Part model, mm, in its own coordinate system. Face numbers are marked on the shaded views. A direction names the side the tool comes from. Coordinates: 2 decimals unless noted, no trailing zeros. Loops run counter-clockwise (first coordinate to the right, second up) from the corner with the lowest first, then second, coordinate; pieces in that order, holes last. Notation, with made-up numbers: (39.25, 70) - (50.25, 70) arc R30 ccw to (50.25, 108) - close; hole circle Ø6 at (-5.75, 81.25). An arc over 180 degrees is marked (long way). Answer as CSV lines item,"result".
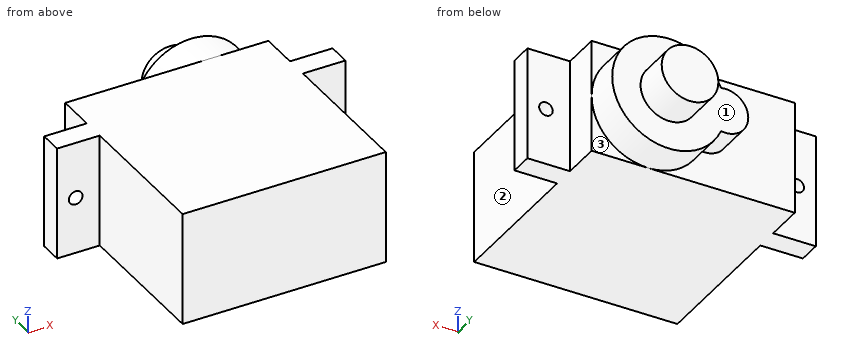
from build123d import *

# Parameters (mm, degrees)
SKETCH_1_W          = 22.4
SKETCH_1_H          = 12.5
EXTRUDE_1_DEPTH     = 22.8
EXTRUDE_START       = 16.1
SKETCH_2_W          = 31.8
SKETCH_2_H          = 12.5
EXTRUDE_2_DEPTH     = 2.5
CUT_EXTRUDE_1_REACH = 27.255
SKETCH_3_R          = 0.75
EXTRUDE_3_DEPTH     = 4
SKETCH_6_R          = 3.125
EXTRUDE_4_DEPTH     = 4.1


with BuildPart() as part:
    # 草图1 → 凸台-拉伸1 (new body)
    with BuildSketch(Plane(origin=(0, 0, 0), x_dir=(1, 0, 0), z_dir=(0, 1, 0))):
        Rectangle(SKETCH_1_W, SKETCH_1_H)
    extrude(amount=EXTRUDE_1_DEPTH)

    # 草图2 → 凸台-拉伸2 (add)
    with BuildSketch(Plane(origin=(0, 0, 0), x_dir=(1, 0, 0), z_dir=(0, 1, 0)).offset(EXTRUDE_START)):
        Rectangle(SKETCH_2_W, SKETCH_2_H)
    extrude(amount=EXTRUDE_2_DEPTH)

    # 草图3 → 切除-拉伸1 (cut, up to next)
    with BuildSketch(Plane(origin=(0, 18.6, 0), x_dir=(1, 0, 0), z_dir=(0, 1, 0)), mode=Mode.PRIVATE) as cut_extrude_1_sk1:
        with Locations(Location((-13.85, 0, 0), (0, 0, 270))):
            Circle(SKETCH_3_R)
    cut_extrude_1_tool1 = extrude(cut_extrude_1_sk1.sketch, amount=-CUT_EXTRUDE_1_REACH, mode=Mode.PRIVATE) & part.part
    # 草图3 → 切除-拉伸1 (cut, up to next)
    with BuildSketch(Plane(origin=(0, 18.6, 0), x_dir=(1, 0, 0), z_dir=(0, 1, 0)), mode=Mode.PRIVATE) as cut_extrude_1_sk2:
        with Locations(Location((13.85, 0, 0), (0, 0, 270))):
            Circle(SKETCH_3_R)
    cut_extrude_1_tool2 = extrude(cut_extrude_1_sk2.sketch, amount=-CUT_EXTRUDE_1_REACH, mode=Mode.PRIVATE) & part.part
    add(cut_extrude_1_tool1.solids().sort_by_distance((-13.85, 18.6, 0))[0], mode=Mode.SUBTRACT)
    add(cut_extrude_1_tool2.solids().sort_by_distance((13.85, 18.6, 0))[0], mode=Mode.SUBTRACT)

    # 草图4 → 凸台-拉伸3 (add)
    with BuildSketch(Plane(origin=(0, 22.8, 0), x_dir=(1, 0, 0), z_dir=(0, 1, 0))):
        with BuildLine():
            ThreePointArc((-0.8, -2.449489743), (11.2, 0), (-0.8, 2.449489743))
            ThreePointArc((-0.8, 2.449489743), (-3.8, 0), (-0.8, -2.449489743))
        make_face()
    extrude(amount=EXTRUDE_3_DEPTH)

    # 草图6 → 凸台-拉伸4 (add)
    with BuildSketch(Plane(origin=(0, 26.8, 0), x_dir=(1, 0, 0), z_dir=(0, 1, 0))):
        with Locations(Location((4.95, 0, 0), (0, 0, 270))):
            Circle(SKETCH_6_R)
    extrude(amount=EXTRUDE_4_DEPTH)


solid = part.part
Q1. Saw through at B-B (x = -1.3). Give the cut face in (y, z), then the cut area to 3 significant figures.
Results:
outline,"(0, -6.25) - (22.8, -6.25) - (22.8, -2.5) - (26.8, -2.5) - (26.8, 2.5) - (22.8, 2.5) - (22.8, 6.25) - (0, 6.25) - close"
area,"305 mm^2"
Q2. Flat gauge pins, fed straight in: pin 1 (2.5 mm diameter, centred on x = 14, z = 2.5, fed in from -Y); pin 2 (1.5 mm diameter, centred on x = -12, y = 22, fed in from +Z); pin 3 (5 mm diameter, centred on x = -14, z = 3, fed in from +Y); pin 4 (1.9 mm diameter, centred on x = 9, z = -4, fed in from +Y). Where does each tip first touch, or does it go through?
Results:
pin 1,"stops at y = 16.1"
pin 2,"passes through"
pin 3,"stops at y = 18.6"
pin 4,"stops at y = 26.8"
Q3. Saw through at C-C (z = 1.5). Give the cut face in (x, y), then the cut area to 3 significant figures.
Results:
outline,"(-15.9, 16.1) - (-11.2, 16.1) - (-11.2, 0) - (11.2, 0) - (11.2, 16.1) - (15.9, 16.1) - (15.9, 18.6) - (11.2, 18.6) - (11.2, 22.8) - (11.02, 22.8) - (11.02, 26.8) - (7.69, 26.8) - (7.69, 30.9) - (2.21, 30.9) - (2.21, 26.8) - (-3.3, 26.8) - (-3.3, 22.8) - (-11.2, 22.8) - (-11.2, 18.6) - (-15.9, 18.6) - close"
area,"614 mm^2"
Q4. Which spindle directions (+Z, -Z, +X, -X, +Y, -Y) get a long thin tool onto all of the face, cutting with end or side? Do the marked faces 1, 2 and 3. Say none if no direction does.
Results:
face 1,"+Y"
face 2,"+Z, -Z, +X, -Y"
face 3,"-Z, +X, +Y"
Q5. Saw through at A-A (x = -13.85). Give the cut face in (y, z).
Results:
outline,"(16.1, -6.25) - (18.6, -6.25) - (18.6, -0.75) - (16.1, -0.75) - close; (16.1, 0.75) - (18.6, 0.75) - (18.6, 6.25) - (16.1, 6.25) - close"
Q6. Wall check: L1, parallel to X at y = 17.9, z = 0; L2, parallel to Y at x = -1, z = -5; L3, parallel to X at y = 11, z = 5.25. Give the ranges that are in metal, low to high.
Results:
L1,"x = -15.9 to -14.6, -13.1 to 13.1, 14.6 to 15.9"
L2,"y = 0 to 22.8"
L3,"x = -11.2 to 11.2"
Q7. Saw through at D-D (y = 27.5). Give the cut face in (x, z) (3 decimals), then the cut area to 3 significant figures.
Results:
outline,"circle Ø6.25 at (4.95, 0)"
area,"30.7 mm^2"
